```python
from build123d import *

# Parameters (mm, degrees)
SZKIC1_W                     = 5
SZKIC1_H                     = 10
DODANIE_WYCI_GNI_CIE1_DEPTH  = 1
DODANIE_WYCI_GNI_CIE4_DEPTH  = 4
ZAOKR_GLENIE2_R              = 5
SZKIC3_W                     = 1
SZKIC3_H                     = 4
WYTNIJ_WYCI_GNI_CIE1_DEPTH   = 4
SZKIC4_W                     = 0.5
SZKIC4_H                     = 4
DODANIE_WYCI_GNI_CIE5_DEPTH  = 1
SZKIC5_R                     = 0.25
DODANIE_WYCI_GNI_CIE6_DEPTH  = 2
SZKIC6_R                     = 0.55
SZKIC6_R_2                   = 0.5
DODANIE_WYCI_GNI_CIE7_DEPTH  = 0.5
SZKIC7_W                     = 7
SZKIC7_H                     = 1
DODANIE_WYCI_GNI_CIE8_DEPTH  = 1
SZKIC11_R                    = 0.25
DODANIE_WYCI_GNI_CIE10_DEPTH = 0.5
SZKIC12_R                    = 0.125
WYTNIJ_WYCI_GNI_CIE2_DEPTH   = 1


with BuildPart() as part:
    # Szkic1 → Dodanie-wyciągnięcie1 (new body)
    with BuildSketch(Plane(origin=(0, 0, 0), x_dir=(1, 0, 0), z_dir=(0, 1, 0))):
        Rectangle(SZKIC1_W, SZKIC1_H)
    extrude(amount=DODANIE_WYCI_GNI_CIE1_DEPTH)

    # Szkic2 → Dodanie-wyciągnięcie4 (add)
    with BuildSketch(Plane(origin=(0, 1, 0), x_dir=(1, 0, 0), z_dir=(0, 1, 0))):
        Polygon((-2.5, 5), (2.5, 5), (2.5, 3.5), (-0.5, 3.5), (-0.5, -3.5), (2.5, -3.5), (2.5, -5), (-2.5, -5), align=None)
    extrude(amount=DODANIE_WYCI_GNI_CIE4_DEPTH)

    # Zaokrąglenie2
    zaokr_glenie2_edges = [part.edges().sort_by_distance(p)[0] for p in [
        (-2.5, 2.5, -5),
        (-2.5, 2.5, 5),
    ]]
    fillet(zaokr_glenie2_edges, radius=ZAOKR_GLENIE2_R - 0.0001)  # a hair under: the kernel refuses the full size

    # Szkic3 → Wytnij-wyciągnięcie1 (cut)
    with BuildSketch(Plane(origin=(0, 1, 0), x_dir=(1, 0, 0), z_dir=(0, 1, 0))):
        with Locations((0.5, 0)):
            Rectangle(SZKIC3_W, SZKIC3_H)
    extrude(amount=-WYTNIJ_WYCI_GNI_CIE1_DEPTH, mode=Mode.SUBTRACT)

    # Szkic4 → Dodanie-wyciągnięcie5 (add)
    with BuildSketch(Plane(origin=(0, 1, 0), x_dir=(1, 0, 0), z_dir=(0, 1, 0))):
        with Locations((-0.25, 0)):
            Rectangle(SZKIC4_W, SZKIC4_H)
    extrude(amount=DODANIE_WYCI_GNI_CIE5_DEPTH)

    # Szkic5 → Dodanie-wyciągnięcie6 (add)
    with BuildSketch(Plane(origin=(0, 1, 0), x_dir=(1, 0, 0), z_dir=(0, 1, 0))):
        with Locations(Location((1.75, 0, 0), (0, 0, 90))):
            Circle(SZKIC5_R)
    extrude(amount=DODANIE_WYCI_GNI_CIE6_DEPTH)

    # Szkic6 → Dodanie-wyciągnięcie7 (add)
    with BuildSketch(Plane(origin=(0, 1, 0), x_dir=(1, 0, 0), z_dir=(0, 1, 0))):
        with Locations(Location((1.75, 0, 0), (0, 0, 90))):
            Circle(SZKIC6_R)
        with Locations(Location((1.75, 0, 0), (0, 0, 270))):
            Circle(SZKIC6_R_2, mode=Mode.SUBTRACT)
    extrude(amount=DODANIE_WYCI_GNI_CIE7_DEPTH)

    # Szkic7 → Dodanie-wyciągnięcie8 (add)
    with BuildSketch(Plane(origin=(-0.5, 0, 0), x_dir=(0, 0, -1), z_dir=(1, 0, 0))):
        with Locations((0, 4.5)):
            Rectangle(SZKIC7_W, SZKIC7_H)
    extrude(amount=DODANIE_WYCI_GNI_CIE8_DEPTH)

    # Szkic11 → Dodanie-wyciągnięcie10 (add)
    with BuildSketch(Plane(origin=(2.5, 0, 0), x_dir=(0, 0, -1), z_dir=(1, 0, 0))):
        with Locations(Location((-4.25, 3.503110499, 0), (0, 0, 180))):
            Circle(SZKIC11_R)
        with Locations(Location((-4.25, 1.503110499, 0), (0, 0, 180))):
            Circle(SZKIC11_R)
        with Locations(Location((4.25, 3.503110499, 0), (0, 0, 180))):
            Circle(SZKIC11_R)
        with Locations(Location((4.25, 1.503110499, 0), (0, 0, 180))):
            Circle(SZKIC11_R)
    extrude(amount=DODANIE_WYCI_GNI_CIE10_DEPTH)

    # Szkic12 → Wytnij-wyciągnięcie2 (cut)
    with BuildSketch(Plane(origin=(0, 0, 0), x_dir=(0, 0, -1), z_dir=(1, 0, 0))):
        with Locations((0, 1.5)):
            Circle(SZKIC12_R)
    extrude(amount=-WYTNIJ_WYCI_GNI_CIE2_DEPTH, mode=Mode.SUBTRACT)


solid = part.part
```
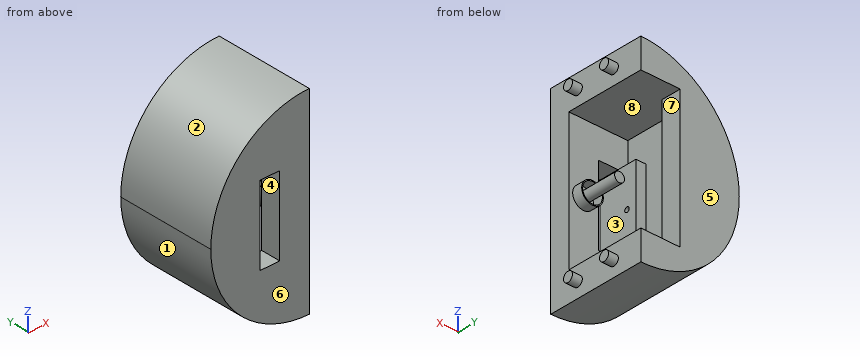
Work out the finished part from the listing and answer in its coordinate system (mm). Face numbers are marked on the shaded views. A direction names the side the tool comes from. Round coordinates to 2 decimals unless told otherwise and drop trailing zeros. Write each loop counter-clockwise with the first axis right and the second up, starting at its lowest first coordinate (ties: lowest second). Pieces come first, ordered by that corner, then holes. Notation, with made-up numbers: (68.5, 75.5) - (91.5, 75.5) arc R20 cw to (91.5, 111.5) - close; hole circle Ø3 at (49.5, 54.25). An arc over 180 degrees is marked (long way). Return JSON: item names as keys, results as strings. Group by question number.
Q1. The part is cut by section D-D on x = 1.75. Write down the section's boundary in (y, z).
Q2. The part is cut by section A-A on z = -1.25. Write down the section's boundary in (x, y).
Q3. The mould has two halves that part along Z. Classify the marked faces 1, 2 and 3: released by +Z, released by -Z, zero draft, split by the parting line, or undercut.
Q4. Each of these flat-tipped pins is pushed along its axis until it touches: pin 1 Ø0.9 at (y, z) = (2, 0.5) entering from +X; pin 2 Ø0.6 at (x, z) = (1.5, 0) entering from +Y; pin 3 Ø0.8 at (x, y) = (0.5, 0.5) entering from -Z. Where does it stop, or does it pass through?
Q5. Find the intervals of material crossed by L1, parallel to Y at x = -0.3, z = 0 (3 decimals); L2, parallel to Y at x = -0.55, z = 0 (3 decimals); L3, parallel to Y at x = 0.35, z = 0.5, in increasing order.
Q6. For the marked faces 4, 5, 6, 7 and 8, determine the directions among +Z, -Z, +X, -X, +Y, -Y from which every point of the face is accessible in a straight line to the end or side of a thin tool.
Q7. The part is cut by section C-C on x = -0.4. Write down the section's boundary in (y, z) (3 decimals).
Solved:
{
 "1": {"outline": "(0, -4.94) - (5, -4.94) - (5, -3.5) - (1, -3.5) - (1, -0.55) - (1.5, -0.55) - (1.5, -0.5) - (1, -0.5) - (1, -0.25) - (3, -0.25) - (3, 0.25) - (1, 0.25) - (1, 0.5) - (1.5, 0.5) - (1.5, 0.55) - (1, 0.55) - (1, 3.5) - (5, 3.5) - (5, 4.94) - (0, 4.94) - close"},
 "2": {"outline": "(-2.34, 0) - (0, 0) - (0, 2) - (-0.5, 2) - (-0.5, 4) - (0.5, 4) - (0.5, 5) - (-2.34, 5) - close; (1, 0) - (2.5, 0) - (2.5, 1) - (1, 1) - close"},
 "3": {"face 1": "released by -Z", "face 2": "released by +Z", "face 3": "undercut"},
 "4": {"pin 1": "x = 1.99", "pin 2": "y = 3", "pin 3": "z = -4.74"},
 "5": {"L1": "0 to 1.375, 1.625 to 2, 4 to 5", "L2": "0 to 1.375, 1.625 to 5", "L3": "4 to 5"},
 "6": {"face 4": "+Y, -Y", "face 5": "+Z, -Z, +X, -X, +Y", "face 6": "+Z, -Z, +X, -X, -Y", "face 7": "+X, +Y", "face 8": "+X"},
 "7": {"outline": "(0, -4.073) - (5, -4.073) - (5, 4.073) - (0, 4.073) - close; hole (1, -3.5) - (4, -3.5) - (4, 3.5) - (1, 3.5) - (1, 2) - (2, 2) - (2, -2) - (1, -2) - close; hole circle Ø0.25 at (1.5, 0)"}
}
